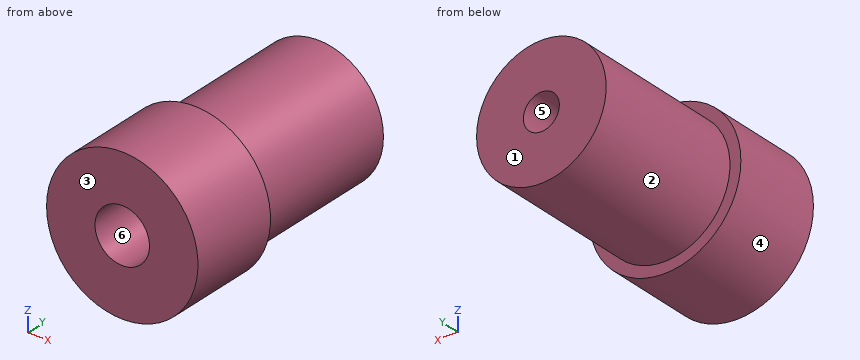
Autodesk Inventor part; units mm, degrees
ref_plane "YZ Plane" through (0, 0, 0) normal (1, 0, 0) x (0, 1, 0)
ref_plane "XZ Plane" through (0, 0, 0) normal (0, 1, 0) x (-1, 0, 0)
ref_plane "XY Plane" through (0, 0, 0) normal (0, 0, 1) x (1, 0, 0)
sketch "Esquisse1" plane through (0, 0, 0) normal (0, 1, 0) x (-1, 0, 0)
  circle A0 centre (0, 0) radius 6.95
  circle A1 centre (0, 0) radius 2.5
  dimension "d0" = 13.9
  dimension "d1" = 5
extrude "Extrusion1" add sketch "Esquisse1" along normal blind 8.5
sketch "Esquisse2" plane through (0, 8.5, 0) normal (0, 1, 0) x (1, 0, 0)
  circle A0 centre (0, 0) radius 5.95
  circle A1 centre (0, 0) radius 2.5
  dimension "d4" = 11.9
extrude "Extrusion2" add sketch "Esquisse2" along normal blind 9.5
sketch "Esquisse3" plane through (0, 18, 0) normal (0, 1, 0) x (1, 0, 0)
  circle A0 centre (0, 0) radius 5.95
  circle A1 centre (0, 0) radius 1.65
  dimension "d3" = 0
  dimension "d7" = 3.3
extrude "Extrusion3" add sketch "Esquisse3" along normal blind 5
thread "Filetage1"
properties part number "moyeu"
CAD build for the part. Positions are in the model's coordinates, mm. Face numbers are marked on the shaded views. A direction names the side the tool comes from. Give positions to 0.01 mm unless a question says otherwise; leave off trailing zeros. Write each loop counter-clockwise with the first axis right and the second up, starting at its lowest first coordinate (ties: lowest second). Pieces come first, ordered by that corner, then holes. Notation, with made-up numbers: (-31.75, 33.25) -> (6.25, 33.25) arc R18 cw to (6.25, 53.25) -> close; hole circle Ø1 at (73, 71). An arc over 180 degrees is marked (long way). Write each question's results on one line, items separated by ' | '.
1. Cut at C-C, the plane z = -3.75. Write the cut outline in (x, y), then the cut area to 3 significant figures.
Geometry check:
outline: (-5.85, 0) -> (5.85, 0) -> (5.85, 8.5) -> (4.62, 8.5) -> (4.62, 23) -> (-4.62, 23) -> (-4.62, 8.5) -> (-5.85, 8.5) -> close | area: 233 mm²
2. Two-plate mould, pull along Z, no slides. Class the marked faces 3, 4, 5 and 6: pulls with the +Z half, pulls with the -Z half, needs draft (parallel to the pull), parting line crosses it, or undercut.
Geometry check:
face 3: needs draft | face 4: parting line crosses it | face 5: undercut | face 6: undercut
3. Which spindle directions (+Z, -Z, +X, -X, +Y, -Y) get a long thin tool onto all of the face, cutting with end or side? Do the marked faces 1 and 2. Say none if no direction does.
Geometry check:
face 1: +Z, -Z, +X, -X, +Y | face 2: +Y
4. Cut at A-A, the plane y = 6.25. Write the cut outline in (x, z), then the cut area to 3 significant figures.
Geometry check:
outline: circle Ø13.9 at (0, 0); hole circle Ø5 at (0, 0) | area: 132 mm²
5. Drop flat-ended pins along their axis: P1, Ø2, axis at x = 3, y = 20, coming from the -Z side; P2, Ø8, axis at x = -5.5, y = 15, coming from the -Z side; P3, Ø3, axis at y = 7.5, z = 3.5, coming from the +X side; P4, Ø2.5, axis at x = 0, z = 0, coming from the -Y side. Give the stop position or say it passes through.
Geometry check:
P1: z = -5.6 | P2: z = -5.76 | P3: x = 6.66 | P4: through
6. Wall check: probe 1 along X at (y, z) = (21.6, 0); probe 2 along Z at (x, y) = (0, 9). Give the ranges that are in metal, low to high. Write a range as [from, to].
Geometry check:
probe 1: [-5.95, -1.65], [1.65, 5.95] | probe 2: [-5.95, -2.5], [2.5, 5.95]
7. Cut at D-D, the plane y = 20.25. Write the cut outline in (x, z).
Geometry check:
outline: circle Ø11.9 at (0, 0); hole circle Ø3.3 at (0, 0)
